Verification items for the finished model (mm, model axes). A direction names the side the tool comes from. Round coordinates to 2 decimals unless told otherwise and drop trailing zeros. Loops run counter-clockwise (first coordinate to the right, second up) from the corner with the lowest first, then second, coordinate; pieces in that order, holes last. Notation, with made-up numbers: M 35,13 L 67,13 A27 ccw 67,45 Z; hole C -1.5,11.5 d8. An arc over 180 degrees is marked long. One line per item, written item: value.
from build123d import *

# Parameters (mm, degrees)
SKETCH1_R                           = 7
BOSS_EXTRUDE1_DEPTH                 = 4.5
SKETCH2_R                           = 2
CUT_EXTRUDE1_DEPTH                  = 4
CUT_EXTRUDE1_DIRECTION_2_REACH      = 84.52
CUT_EXTRUDE1_DIRECTION_2_END_RADIUS = 35
CUT_EXTRUDE2_REACH                  = 85.44
CUT_EXTRUDE3_DEPTH                  = 84.439778024
CUT_EXTRUDE3_DEPTH_BACK             = 84.439778024
FILLET1_R                           = 1


with BuildPart() as part:
    # Sketch1 → Boss-Extrude1 (new, symmetric)
    # profile 1 of 2: a face of its own
    with BuildSketch(Plane(origin=(0, 0, 0), x_dir=(1, 0, 0), z_dir=(0, 1, 0))):
        with BuildLine():
            Line((-1.254341559, 11.934262744), (-28.287114055, 9.093003864))
            ThreePointArc((-28.287114055, 9.093003864), (-43.847711602, 9.487707298), (-58.78314626, 13.871858114))
            ThreePointArc((-58.78314626, 13.871858114), (-66.945926578, 15.925337372), (-75.327562788, 15.153369736))
            Line((-75.327562788, 15.153369736), (-69.509618943, 5.076395401))
            Line((-69.509618943, 5.076395401), (-62.581415713, 9.076395401))
            Line((-62.581415713, 9.076395401), (-56.581415713, -1.315909444))
            Line((-56.581415713, -1.315909444), (-63.509618943, -5.315909444))
            Line((-63.509618943, -5.315909444), (-61.251109949, -9.227761772))
            ThreePointArc((-61.251109949, -9.227761772), (-53.508040015, -7.353839298), (-45.541787079, -7.279464651))
            Line((-45.541787079, -7.279464651), (-1.254341559, -11.934262744))
            ThreePointArc((-1.254341559, -11.934262744), (12, 0), (-1.254341559, 11.934262744))
        make_face()
        with Locations(Location((0, 0, 0), (0, 0, 270))):
            Circle(SKETCH1_R, mode=Mode.SUBTRACT)
    # profile 2 of 2: a face of its own
    with BuildSketch(Plane(origin=(0, 0, 0), x_dir=(1, 0, 0), z_dir=(0, 1, 0))):
        with BuildLine():
            Line((-69.509618943, 5.076395401), (-75.327562788, 15.153369736))
            ThreePointArc((-75.327562788, 15.153369736), (-82.282399056, 12.101775932), (-88, 7.102674843))
            Line((-88, 7.102674843), (-86.5, 4.504598631))
            Line((-86.5, 4.504598631), (-81.303847577, 7.504598631))
            Line((-81.303847577, 7.504598631), (-76.107695155, 4.504598631))
            Line((-76.107695155, 4.504598631), (-66.705771366, -11.78001106))
            ThreePointArc((-66.705771366, -11.78001106), (-64.033436336, -10.386349776), (-61.251109949, -9.227761772))
            Line((-61.251109949, -9.227761772), (-63.509618943, -5.315909444))
            Line((-63.509618943, -5.315909444), (-69.509618943, 5.076395401))
        make_face()
    extrude(amount=BOSS_EXTRUDE1_DEPTH, both=True)

    # Sketch2 → Cut-Extrude1 (cut)
    with BuildSketch(Plane(origin=(-19.575548424, 0, -33.905844457), x_dir=(0.8660254037844372, 0, -0.5000000000000027), z_dir=(0.5000000000000027, 0, 0.8660254037844372))):
        with Locations(Location((-53.658898112, 0, 0), (0, 0, 180))):
            Circle(SKETCH2_R)
    extrude(amount=-CUT_EXTRUDE1_DEPTH, mode=Mode.SUBTRACT)

    # Cut-Extrude1 direction 2: up to this cylinder (the profile starts outside it)
    cut_extrude1_direction_2_end = Plane(origin=(-49.200283293, 0, 42.087730989), z_dir=(0, -1, 0)) * Cylinder(CUT_EXTRUDE1_DIRECTION_2_END_RADIUS, 240.04, mode=Mode.PRIVATE)
    # Sketch2 → Cut-Extrude1 direction 2 (cut, up to the surface)
    with BuildSketch(Plane(origin=(-19.575548424, 0, -33.905844457), x_dir=(0.8660254037844372, 0, -0.5000000000000027), z_dir=(0.5000000000000027, 0, 0.8660254037844372)), mode=Mode.PRIVATE) as cut_extrude1_direction_2_sk1:
        with Locations(Location((-53.658898112, 0, 0), (0, 0, 180))):
            Circle(SKETCH2_R)
    cut_extrude1_direction_2_tool1 = extrude(cut_extrude1_direction_2_sk1.sketch, amount=CUT_EXTRUDE1_DIRECTION_2_REACH, mode=Mode.PRIVATE) - cut_extrude1_direction_2_end
    add(cut_extrude1_direction_2_tool1.solids().sort_by_distance((-66.045517, 0, -7.076395))[0], mode=Mode.SUBTRACT)

    # Sketch3 → Cut-Extrude2 (cut, up to next)
    with BuildSketch(Plane(origin=(-23.575548424, 0, -40.834047687), x_dir=(0.8660254037844374, 0, -0.5000000000000023), z_dir=(0.5000000000000023, 0, 0.8660254037844374)), mode=Mode.PRIVATE) as cut_extrude2_sk1:
        with BuildLine():
            ThreePointArc((-62.220147611, 1.25), (-62.546025426, 0.662382443), (-62.658898112, 0))
            Line((-62.658898112, 0), (-58.658898112, 0))
            ThreePointArc((-58.658898112, 0), (-58.771770798, 0.662382443), (-59.097648612, 1.25))
            ThreePointArc((-59.097648612, 1.25), (-60.658898112, 2), (-62.220147611, 1.25))
        make_face()
    cut_extrude2_tool1 = extrude(cut_extrude2_sk1.sketch, amount=CUT_EXTRUDE2_REACH, mode=Mode.PRIVATE) & part.part
    # Sketch3 → Cut-Extrude2 (cut, up to next)
    with BuildSketch(Plane(origin=(-23.575548424, 0, -40.834047687), x_dir=(0.8660254037844374, 0, -0.5000000000000023), z_dir=(0.5000000000000023, 0, 0.8660254037844374)), mode=Mode.PRIVATE) as cut_extrude2_sk2:
        with BuildLine():
            Line((-58.658898112, 0), (-62.658898112, 0))
            ThreePointArc((-62.658898112, 0), (-62.546025426, -0.662382443), (-62.220147611, -1.25))
            ThreePointArc((-62.220147611, -1.25), (-60.658898112, -2), (-59.097648612, -1.25))
            ThreePointArc((-59.097648612, -1.25), (-58.771770798, -0.662382443), (-58.658898112, 0))
        make_face()
    cut_extrude2_tool2 = extrude(cut_extrude2_sk2.sketch, amount=CUT_EXTRUDE2_REACH, mode=Mode.PRIVATE) & part.part
    # Sketch3 → Cut-Extrude2 (cut, up to next)
    with BuildSketch(Plane(origin=(-23.575548424, 0, -40.834047687), x_dir=(0.8660254037844374, 0, -0.5000000000000023), z_dir=(0.5000000000000023, 0, 0.8660254037844374)), mode=Mode.PRIVATE) as cut_extrude2_sk3:
        with BuildLine():
            ThreePointArc((-62.220147611, 1.25), (-62.546025426, 0.662382443), (-62.658898112, 0))
            Line((-62.658898112, 0), (-58.658898112, 0))
            ThreePointArc((-58.658898112, 0), (-58.771770798, 0.662382443), (-59.097648612, 1.25))
            ThreePointArc((-59.097648612, 1.25), (-60.658898112, 2), (-62.220147611, 1.25))
        make_face()
    cut_extrude2_tool3 = extrude(cut_extrude2_sk3.sketch, amount=CUT_EXTRUDE2_REACH, mode=Mode.PRIVATE) & part.part
    # Sketch3 → Cut-Extrude2 (cut, up to next)
    with BuildSketch(Plane(origin=(-23.575548424, 0, -40.834047687), x_dir=(0.8660254037844374, 0, -0.5000000000000023), z_dir=(0.5000000000000023, 0, 0.8660254037844374)), mode=Mode.PRIVATE) as cut_extrude2_sk4:
        with BuildLine():
            Line((-58.658898112, 0), (-62.658898112, 0))
            ThreePointArc((-62.658898112, 0), (-62.546025426, -0.662382443), (-62.220147611, -1.25))
            ThreePointArc((-62.220147611, -1.25), (-60.658898112, -2), (-59.097648612, -1.25))
            ThreePointArc((-59.097648612, -1.25), (-58.771770798, -0.662382443), (-58.658898112, 0))
        make_face()
    cut_extrude2_tool4 = extrude(cut_extrude2_sk4.sketch, amount=CUT_EXTRUDE2_REACH, mode=Mode.PRIVATE) & part.part
    # Sketch3 → Cut-Extrude2 (cut, up to next)
    with BuildSketch(Plane(origin=(-23.575548424, 0, -40.834047687), x_dir=(0.8660254037844374, 0, -0.5000000000000023), z_dir=(0.5000000000000023, 0, 0.8660254037844374)), mode=Mode.PRIVATE) as cut_extrude2_sk5:
        with BuildLine():
            Line((-66.658898112, 1.25), (-66.658898112, 0))
            Line((-66.658898112, 0), (-62.658898112, 0))
            ThreePointArc((-62.658898112, 0), (-62.546025426, 0.662382443), (-62.220147611, 1.25))
            Line((-62.220147611, 1.25), (-66.658898112, 1.25))
        make_face()
    cut_extrude2_tool5 = extrude(cut_extrude2_sk5.sketch, amount=CUT_EXTRUDE2_REACH, mode=Mode.PRIVATE) & part.part
    # Sketch3 → Cut-Extrude2 (cut, up to next)
    with BuildSketch(Plane(origin=(-23.575548424, 0, -40.834047687), x_dir=(0.8660254037844374, 0, -0.5000000000000023), z_dir=(0.5000000000000023, 0, 0.8660254037844374)), mode=Mode.PRIVATE) as cut_extrude2_sk6:
        with BuildLine():
            Line((-62.658898112, 0), (-66.658898112, 0))
            Line((-66.658898112, 0), (-66.658898112, -1.25))
            Line((-66.658898112, -1.25), (-62.220147611, -1.25))
            ThreePointArc((-62.220147611, -1.25), (-62.546025426, -0.662382443), (-62.658898112, 0))
        make_face()
    cut_extrude2_tool6 = extrude(cut_extrude2_sk6.sketch, amount=CUT_EXTRUDE2_REACH, mode=Mode.PRIVATE) & part.part
    # Sketch3 → Cut-Extrude2 (cut, up to next)
    with BuildSketch(Plane(origin=(-23.575548424, 0, -40.834047687), x_dir=(0.8660254037844374, 0, -0.5000000000000023), z_dir=(0.5000000000000023, 0, 0.8660254037844374)), mode=Mode.PRIVATE) as cut_extrude2_sk7:
        with BuildLine():
            ThreePointArc((-59.097648612, 1.25), (-58.771770798, 0.662382443), (-58.658898112, 0))
            Line((-58.658898112, 0), (-57.658898112, 0))
            Line((-57.658898112, 0), (-57.658898112, 1.25))
            Line((-57.658898112, 1.25), (-59.097648612, 1.25))
        make_face()
    cut_extrude2_tool7 = extrude(cut_extrude2_sk7.sketch, amount=CUT_EXTRUDE2_REACH, mode=Mode.PRIVATE) & part.part
    # Sketch3 → Cut-Extrude2 (cut, up to next)
    with BuildSketch(Plane(origin=(-23.575548424, 0, -40.834047687), x_dir=(0.8660254037844374, 0, -0.5000000000000023), z_dir=(0.5000000000000023, 0, 0.8660254037844374)), mode=Mode.PRIVATE) as cut_extrude2_sk8:
        with BuildLine():
            Line((-57.658898112, 0), (-58.658898112, 0))
            ThreePointArc((-58.658898112, 0), (-58.771770798, -0.662382443), (-59.097648612, -1.25))
            Line((-59.097648612, -1.25), (-57.658898112, -1.25))
            Line((-57.658898112, -1.25), (-57.658898112, 0))
        make_face()
    cut_extrude2_tool8 = extrude(cut_extrude2_sk8.sketch, amount=CUT_EXTRUDE2_REACH, mode=Mode.PRIVATE) & part.part
    add(cut_extrude2_tool1.solids().sort_by_distance((-76.107695, 0.848826, -10.504599))[0], mode=Mode.SUBTRACT)
    add(cut_extrude2_tool2.solids().sort_by_distance((-76.107695, -0.848826, -10.504599))[0], mode=Mode.SUBTRACT)
    add(cut_extrude2_tool3.solids().sort_by_distance((-76.107695, 0.848826, -10.504599))[0], mode=Mode.SUBTRACT)
    add(cut_extrude2_tool4.solids().sort_by_distance((-76.107695, -0.848826, -10.504599))[0], mode=Mode.SUBTRACT)
    add(cut_extrude2_tool5.solids().sort_by_distance((-79.509815, 0.635751, -8.540384))[0], mode=Mode.SUBTRACT)
    add(cut_extrude2_tool6.solids().sort_by_distance((-79.509815, -0.635751, -8.540384))[0], mode=Mode.SUBTRACT)
    add(cut_extrude2_tool7.solids().sort_by_distance((-74.009148, 0.664064, -11.716195))[0], mode=Mode.SUBTRACT)
    add(cut_extrude2_tool8.solids().sort_by_distance((-74.009148, -0.664064, -11.716195))[0], mode=Mode.SUBTRACT)

    # Sketch4 → Cut-Extrude3 (cut, two sides: drawn at the far end of the back side and taken through both)
    with BuildSketch(Plane(origin=(-23.575548424, 0, -40.834047687), x_dir=(0.8660254037844374, 0, -0.5000000000000023), z_dir=(0.5000000000000023, 0, 0.8660254037844374)).offset(-CUT_EXTRUDE3_DEPTH_BACK)):
        Polygon((-57.658898112, 4.5), (-72.658898112, 4.5), (-72.658898112, 2), align=None)
        Polygon((-57.658898112, -4.5), (-72.658898112, -4.5), (-72.658898112, -2), align=None)
    extrude(amount=CUT_EXTRUDE3_DEPTH + CUT_EXTRUDE3_DEPTH_BACK, mode=Mode.SUBTRACT)

    # Fillet1
    fillet1_edges = [part.edges().sort_by_distance(p)[0] for p in [
        (-56.581415713, 0, 1.315909444),
        (-62.581415713, 0, -9.076395401),
    ]]
    fillet(fillet1_edges, radius=FILLET1_R)


solid = part.part
(1) Thickness scan on L1, parallel to X at y = 0.75, z = 5.25; L2, parallel to X at y = 1.5, z = -0.75; L3, parallel to Z at x = -58, y = -4. Record the ranges inside material, lowest first. Write a range as from..to.
Completed:
L1: x = -63.4..-61.07, -56.79..-4.63, 4.63..10.79
L2: x = -73.94..-72, -68.95..-67.01, -57.77..-6.96, 6.96..11.98
L3: z = -13.53..-1.14, 2.13..8.21
(2) Sectioned sample at A-A on x = 0. Enter the section's corners in (y, z), and give its area (3 significant figures).
Completed:
outline: M -4.5,-12 L 4.5,-12 L 4.5,-7 L -4.5,-7 Z; M -4.5,7 L 4.5,7 L 4.5,12 L -4.5,12 Z
area: 90.0 mm^2
(3) Sectioned sample at B-B on z = -0.75. Count the separate pieces of the cut face and the enclosed holes in it, and give its area (3 significant figures).
Completed:
separate pieces: 4
enclosed holes: 0
area: 537 mm^2
(4) Mould release check, pull along X, two halves, no side actions. Record for faces 1 (the face through (-43.632, 0.063, -9.454)), 2 (the face through (-14.581, 0.063, -10.534)), 3 (the face through (-71.473, 2.391, 3.524)): +X half, -X half, draft (parallel to the pull), parting line (faces both ways), or undercut.
Completed:
face 1: undercut
face 2: undercut
face 3: -X half
(5) Depth check by flat-ended pin: pin 1 Ø6 at (x, z) = (-1, 2) entering from -Y; pin 2 Ø4 at (x, y) = (-65, 0.5) entering from -Z; pin 3 Ø3 at (x, y) = (-58, 2.5) entering from -Z; pin 4 Ø4 at (x, z) = (-71, 2) entering from +Y. Enter the tip coordinate at first touch or a pass-through.
Completed:
pin 1: passes through
pin 2: stops at z = -15.93
pin 3: stops at z = -14.17
pin 4: stops at y = 4.03
(6) Tool access check on faces 4 (the face through (-67.868, 1.063, -6.024)), 5 (the face through (-73.9, 1.25, -1.2)), 6 (the face through (-68.021, -0.028, -10.554)), 7 (the face through (-78.7, -2.4, -6)). Record the directions out of +Z, -Z, +X, -X, +Y, -Y that give a thin tool (end or side, any length) a straight path to the whole face; none if there is none.
Completed:
face 4: +Y, -Y
face 5: +Z
face 6: none
face 7: +Z, +Y, -Y
